from build123d import *

# Parameters (mm, degrees)
F0_R          = 100
F1_DEPTH      = 15
F1_DEPTH_BACK = 15
F2_R          = 96.202365
F3_DEPTH      = 25
F4_R          = 2.5
F5_R          = 2.5
F6_R          = 17.5
F7_DEPTH      = 30.001
F8_R          = 100
F8_R_2        = 93.75
F9_DEPTH      = 3
F10_R         = 2.5


with BuildPart() as f1:
    # F0 (on Front) → F1 (new body, two sides)
    with BuildSketch(Plane.XZ) as f1_sk:
        Circle(F0_R)
    extrude(amount=F1_DEPTH)
    extrude(f1_sk.sketch, amount=-F1_DEPTH_BACK)

    # F2 (on face) → F3 (cut)
    with BuildSketch(Plane(origin=(0, 15, 0), x_dir=(-1, 0, 0), z_dir=(0, 1, 0))):
        Circle(F2_R)
    extrude(amount=-F3_DEPTH, mode=Mode.SUBTRACT)

    # F4
    f4_edges = [f1.edges().sort_by_distance(p)[0] for p in [
        (96.202365, -10, 0),
    ]]
    fillet(f4_edges, radius=F4_R)

    # F5
    f5_edges = [f1.edges().sort_by_distance(p)[0] for p in [
        (-100, -15, 0),
    ]]
    fillet(f5_edges, radius=F5_R)

    # F6 (on face) → F7 (cut, through all)
    with BuildSketch(Plane.XZ.offset(15)):
        Circle(F6_R)
    extrude(amount=-F7_DEPTH, mode=Mode.SUBTRACT)

    # F8 (on face) → F9 (join)
    with BuildSketch(Plane(origin=(0, 15, 0), x_dir=(-1, 0, 0), z_dir=(0, 1, 0))):
        Circle(F8_R)
        Circle(F8_R_2, mode=Mode.SUBTRACT)
    extrude(amount=F9_DEPTH)

    # F10
    f10_edges = [f1.edges().sort_by_distance(p)[0] for p in [
        (100, 18, 0),
    ]]
    fillet(f10_edges, radius=F10_R)


solid = f1.part
Can you work these out from the model? Positions are in its coordinate system, mm. A direction names the side the tool comes from. Give positions to 0.01 mm unless a question says otherwise; leave off trailing zeros. Loops run counter-clockwise (first coordinate to the right, second up) from the corner with the lowest first, then second, coordinate; pieces in that order, holes last. Notation, with made-up numbers: M 13,54.5 L 70,54.5 A22 ccw 70,60.5 Z; hole C 50,28 d5. An arc over 180 degrees is marked long. One line per item, written item: value.
1) Imagine slicing it at B-B on z = 0. Write out the boundary of the cut face in (x, y), and give its area (3 significant figures).
Geometry check:
outline: M -100,-12.5 A2.5 ccw -97.5,-15 L -17.5,-15 L -17.5,-10 L -93.7,-10 A2.5 cw -96.2,-7.5 L -96.2,15 L -93.75,15 L -93.75,18 L -97.5,18 A2.5 ccw -100,15.5 Z; M 17.5,-15 L 97.5,-15 A2.5 ccw 100,-12.5 L 100,15.5 A2.5 ccw 97.5,18 L 93.75,18 L 93.75,15 L 96.2,15 L 96.2,-7.5 A2.5 cw 93.7,-10 L 17.5,-10 Z
area: 1,050 mm²
2) Imagine slicing it at C-C on y = 1.5. Write out the boundary of the cut face in (x, z), and give its area (3 significant figures).
Geometry check:
outline: C 0,0 d200; hole C 0,0 d192.4
area: 2,340 mm²
3) Please list where these lines run through material, in increasing order: line 1 (Z direction, x = 2, y = 13); line 2 (Z direction, x = 0, y = -12); line 3 (Y direction, x = 0.5, z = 18).
Geometry check:
line 1: z = -99.98 to -96.18, 96.18 to 99.98
line 2: z = -100 to -17.5, 17.5 to 100
line 3: y = -15 to -10
4) I'm going to push flat-ended pins straight in: pin 1 (1 mm diameter, centred on x = -29, y = -11.5, fed in from -Z); pin 2 (3 mm diameter, centred on x = -6.5, y = 11.5, fed in from -Z); pin 3 (5 mm diameter, centred on x = -44.5, y = -9, fed in from +Z). Where does each tip first touch, or does it pass through?
Geometry check:
pin 1: stops at z = -95.85
pin 2: stops at z = -99.87
pin 3: stops at z = 90.75
5) Imagine slicing it at A-A on x = 0. Write out the boundary of the cut face in (y, z).
Geometry check:
outline: M -15,-97.5 A2.5 ccw -12.5,-100 L 15.5,-100 A2.5 ccw 18,-97.5 L 18,-93.75 L 15,-93.75 L 15,-96.2 L -7.5,-96.2 A2.5 cw -10,-93.7 L -10,-17.5 L -15,-17.5 Z; M -15,17.5 L -10,17.5 L -10,93.7 A2.5 cw -7.5,96.2 L 15,96.2 L 15,93.75 L 18,93.75 L 18,97.5 A2.5 ccw 15.5,100 L -12.5,100 A2.5 ccw -15,97.5 Z
6) Thinking about a two-plate mould opening in Y: for faces 3 (the face through (-50.4, 16.48, 79.05)), 4 (the face through (-20, -10, 1)), 5 (the face through (-21, 15, -92)), 6 (the face through (-1, -15, -20)), which applies, +Y half, -Y half, draft (parallel to the pull), parting line (faces both ways), or undercut?
Geometry check:
face 3: draft
face 4: +Y half
face 5: undercut
face 6: -Y half
7) On a 3-axis mill with a long thin cutter (end or side, diameter ignored), from which of +Z, -Z, +X, -X, +Y, -Y can I reach the whole of each face in a straight line? I mean faces 1 (the face through (51, 18, 80)), 2 (the face through (20.855, 3.908, -93.915)). Say none if no direction works.
Geometry check:
face 1: +Z, -Z, +X, -X, +Y
face 2: none
